For this review, use the dimensioned drawing (mm, ordinates from the lowest corner) and the shaded views. A direction names the side the tool comes from. Coordinates: 2 decimals unless noted, no trailing zeros. Order: outer loops, then holes, each group sorted by start corner. A loop starts at its lowest first (then second) coordinate and runs counter-clockwise, first axis right, second up. Notation, with made-up numbers: M 13,61.5 L 51,61.5 A12 cw 51,67.5 Z; hole C 34,72.5 d7. An arc over 180 degrees is marked long. One line per item, written item: value.
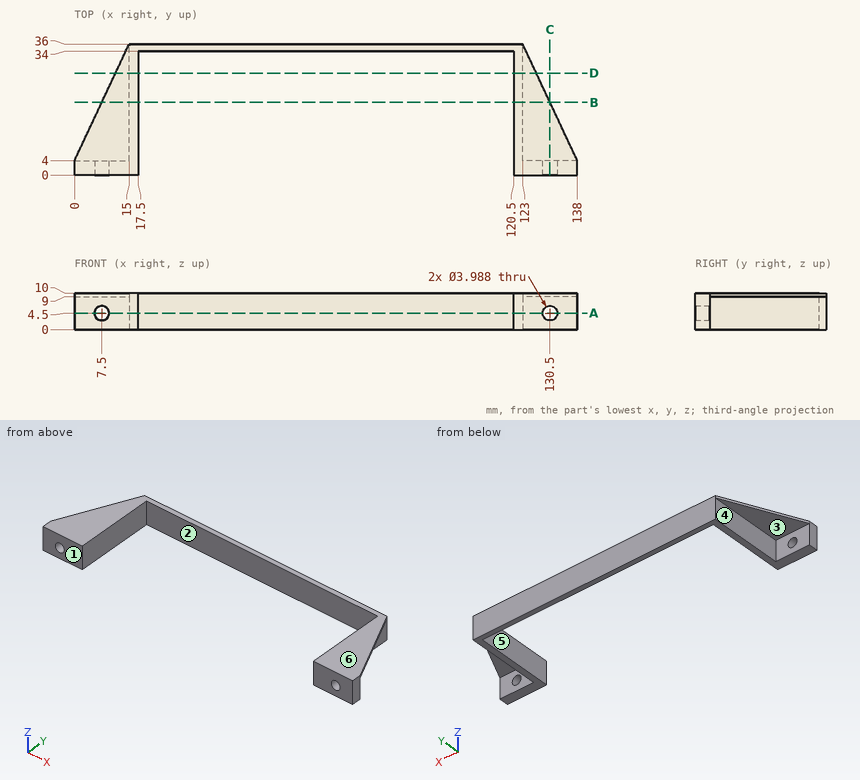
(1) We need section A-A, the plane z = 4.5. State the section outline as (x, y) points.
Geometry results:
outline: M 0,0 L 5.51,0 L 5.51,4 L 0,4 Z; M 9.49,0 L 17.5,0 L 17.5,34 L 120.5,34 L 120.5,0 L 128.51,0 L 128.51,4 L 123,4 L 123,36 L 15,36 L 15,4 L 9.49,4 Z; M 132.49,0 L 138,0 L 138,4 L 132.49,4 Z
(2) Mouldability with a two-part tool opening along X and no side actions: class the marked faces 4, 5 and 6 as +X half, -X half, draft (parallel to the pull), parting line (faces both ways), or undercut.
Geometry results:
face 4: -X half
face 5: undercut
face 6: draft
(3) For L1, parallel to X at y = 1.3, z = 4.5; L2, parallel to Z at x = 130.5, y = 1.75; L3, parallel to X at y = 26, z = 8, list the stretches that pass through material, from the lowest coordinate up.
Geometry results:
L1: x = 0 to 5.51, 9.49 to 17.5, 120.5 to 128.51, 132.49 to 138
L2: z = 0 to 2.51, 6.49 to 10
L3: x = 15 to 17.5, 120.5 to 123
(4) Insertion check: pin 1 Ø3 at (y, z) = (10.5, 5.5) entering from -X; pin 2 Ø4 at (y, z) = (6.5, 5.5) entering from +X; pin 3 Ø7.5 at (x, y) = (8, 12.5) entering from -Z. Each pin has a flat end and moves straight along its axis. Give the tip position at first contact, or say it passes through.
Geometry results:
pin 1: stops at x = 15
pin 2: stops at x = 123
pin 3: stops at z = 9
(5) We need section C-C, the plane x = 130.5. State the section outline as (y, z) points.
Geometry results:
outline: M 0,0 L 4,0 L 4,2.51 L 0,2.51 Z; M 0,6.49 L 4,6.49 L 4,9 L 20,9 L 20,10 L 0,10 Z
(6) We need section D-D, the plane y = 28. State the section outline as (x, z) points.
Geometry results:
outline: M 11.25,9 L 15,9 L 15,0 L 17.5,0 L 17.5,10 L 11.25,10 Z; M 120.5,0 L 123,0 L 123,9 L 126.75,9 L 126.75,10 L 120.5,10 Z
(7) We need section B-B, the plane y = 20. State the section outline as (x, z) points.
Geometry results:
outline: M 7.5,9 L 15,9 L 15,0 L 17.5,0 L 17.5,10 L 7.5,10 Z; M 120.5,0 L 123,0 L 123,9 L 130.5,9 L 130.5,10 L 120.5,10 Z
(8) Tool access review of the marked faces 1, 2 and 3: name each direction out of +Z, -Z, +X, -X, +Y, -Y from which nothing blocks a thin tool from reaching the whole face with its end or side.
Geometry results:
face 1: +Z, -Z, +X, -X, -Y
face 2: +Z, -Z, -Y
face 3: -Z, -X, +Y
